The model under review builds one solid part; all positions refer to its coordinate system, in mm. A direction names the side the tool comes from. Give positions to 0.01 mm unless a question says otherwise; leave off trailing zeros. Loops run counter-clockwise (first coordinate to the right, second up) from the corner with the lowest first, then second, coordinate; pieces in that order, holes last. Notation, with made-up numbers: M 23.25,58.25 L 55.25,58.25 A22 cw 55.25,88.25 Z; hole C 65,53 d9. An arc over 180 degrees is marked long. One line per item, written item: value. Start each with the question number.
Q1. We need section D-D on z = -10. Write out the cut boundary in (x, y).
Q2. For faces 4 (the face through (0, 2, -42)), 5 (the face through (0, 2, -24)), 6 (the face through (0, 2, -7)), 7 (the face through (6, 5, -24)), list the 3-axis set-ups (+Z, -Z, +X, -X, +Y, -Y) from which the entire face can be reached by the end or side of a thin tool; tool diameter is ignored.
Q3. For pin 1 (1.5 mm diameter, centred on y = 3, z = -42.5, fed in from -X), flat-tipped, find the tip position at first contact; note if it passes through.
Q4. We need section C-C on x = -1.75. Write out the cut boundary in (y, z).
Q5. We need section B-B on y = 1.5. Write out the cut boundary in (x, z), plus the area to 3 significant figures.
Q6. We need section A-A on z = -15. Write out the cut boundary in (x, y).
Q7. Mouldability with a two-part tool opening along Z and no side actions: class faces 1 (the face through (11.43, 2.54, -47.4)), 2 (the face through (-4, 2, -15)), 3 (the face through (11.4, 2.54, -0.57)) as released by +Z, released by -Z, zero draft, split by the parting line, or undercut.
Q8. To check wall thickness, follow line 1 along X through (y, z) = (3.2, -33); line 2 along Z through (x, y) = (-0.5, 1.45); line 3 along X through (y, z) = (1.6, -42). State the ranges of each line that lie inside material, in increasing order. Write a range as from..to.
```python
from build123d import *

# Parameters (mm, degrees)
SKETCH1_R           = 1
BOSS_EXTRUDE1_DEPTH = 5
FILLET2_R           = 2


with BuildPart() as part:
    # Sketch1 → Boss-Extrude1 (new body)
    with BuildSketch(Plane(origin=(0, 0, 0), x_dir=(1, 0, 0), z_dir=(0, 1, 0))):
        with BuildLine():
            Line((0, 0), (12, 0))
            Line((12, 0), (12, 48))
            Line((12, 48), (0, 48))
            Line((0, 48), (0, 37))
            ThreePointArc((0, 37), (-4, 33), (0, 29))
            Line((0, 29), (0, 19))
            ThreePointArc((0, 19), (-4, 15), (0, 11))
            Line((0, 11), (0, 0))
        make_face()
        with Locations(Location((0, 33, 0), (0, 0, 270))):
            Circle(SKETCH1_R, mode=Mode.SUBTRACT)
        with Locations(Location((0, 15, 0), (0, 0, 270))):
            Circle(SKETCH1_R, mode=Mode.SUBTRACT)
    extrude(amount=BOSS_EXTRUDE1_DEPTH)

    # Fillet2
    fillet2_edges = [part.edges().sort_by_distance(p)[0] for p in [
        (12, 2.5, 0),
        (0, 2.5, 0),
        (0, 2.5, -48),
        (12, 2.5, -48),
    ]]
    fillet(fillet2_edges, radius=FILLET2_R)


solid = part.part
```
Solved:
1. outline: M 0,0 L 12,0 L 12,5 L 0,5 Z
2. face 4: -Z, -X, +Y, -Y
2. face 5: -X, +Y, -Y
2. face 6: +Z, -X, +Y, -Y
2. face 7: +Z, -Z, +X, -X, +Y
3. pin 1: x = 0
4. outline: M 0,-36.6 L 5,-36.6 L 5,-29.4 L 0,-29.4 Z; M 0,-18.6 L 5,-18.6 L 5,-11.4 L 0,-11.4 Z
5. outline: M 0,-46 A2 ccw 2,-48 L 10,-48 A2 ccw 12,-46 L 12,-2 A2 ccw 10,0 L 2,0 A2 ccw 0,-2 L 0,-11 A4 ccw 0,-19 L 0,-29 A4 ccw 0,-37 Z; hole C 0,-33 d2; hole C 0,-15 d2
5. area: 617 mm2
6. outline: M -4,0 L -1,0 L -1,5 L -4,5 Z; M 1,0 L 12,0 L 12,5 L 1,5 Z
7. face 1: released by -Z
7. face 2: undercut
7. face 3: released by +Z
8. line 1: -4..-1, 1..12
8. line 2: -36.97..-33.87, -32.13..-29.03, -18.97..-15.87, -14.13..-11.03
8. line 3: 0..12
